CAD build for the part. Positions are in the model's coordinates, mm. A direction names the side the tool comes from. Coordinates: 2 decimals unless noted, no trailing zeros. Order: outer loops, then holes, each group sorted by start corner. A loop starts at its lowest first (then second) coordinate and runs counter-clockwise, first axis right, second up. Notation, with made-up numbers: (-8.5, 65) -> (12.5, 65) arc R25 ccw to (12.5, 86) -> close; hole circle Ø4 at (35.25, 75). An arc over 180 degrees is marked (long way). Use one line per item in the form item = value. Start each with the question number.
from build123d import *

# Parameters (mm, degrees)
SKETCH_1_W          = 20
SKETCH_1_H          = 80
SKETCH_1_R          = 1
EXTRUDE_1_DEPTH     = 1.7
SKETCH_2_W          = 8
SKETCH_2_H          = 10
CUT_EXTRUDE_1_DEPTH = 1
SKETCH_3_W          = 5.4
SKETCH_3_H          = 8.7
EXTRUDE_2_DEPTH     = 2


with BuildPart() as part:
    # 草图1 → 凸台-拉伸1 (new body)
    with BuildSketch(Plane(origin=(0, 0, 0), x_dir=(1, 0, 0), z_dir=(0, 1, 0))):
        Rectangle(SKETCH_1_W, SKETCH_1_H)
        with Locations(Location((-5, 15, 0), (0, 0, 270))):
            Circle(SKETCH_1_R, mode=Mode.SUBTRACT)
        with Locations(Location((-5, -15, 0), (0, 0, 270))):
            Circle(SKETCH_1_R, mode=Mode.SUBTRACT)
        with Locations(Location((5, 35, 0), (0, 0, 270))):
            Circle(SKETCH_1_R, mode=Mode.SUBTRACT)
        with Locations(Location((5, -35, 0), (0, 0, 270))):
            Circle(SKETCH_1_R, mode=Mode.SUBTRACT)
    extrude(amount=EXTRUDE_1_DEPTH)

    # 草图2 → 切除-拉伸1 (cut)
    with BuildSketch(Plane(origin=(0, 1.7, 0), x_dir=(1, 0, 0), z_dir=(0, 1, 0))):
        with Locations((-6, -30)):
            Rectangle(SKETCH_2_W, SKETCH_2_H)
        with Locations((-6, 0)):
            Rectangle(SKETCH_2_W, SKETCH_2_H)
        with Locations((-6, 30)):
            Rectangle(SKETCH_2_W, SKETCH_2_H)
    extrude(amount=-CUT_EXTRUDE_1_DEPTH, mode=Mode.SUBTRACT)

    # 草图3 → 凸台-拉伸2 (add)
    with BuildSketch(Plane.XZ):
        with Locations((7.3, 0)):
            Rectangle(SKETCH_3_W, SKETCH_3_H)
    extrude(amount=EXTRUDE_2_DEPTH)


solid = part.part
1) Cut at A-A on x = -5. Give the cut face in (y, z), then the cut area to 3 significant figures.
2) Two-plate mould, pull along X, no slides. Class faces 4 (the face through (-10, 0.5, 0.6)), 5 (the face through (7, -1, 4.35)), 6 (the face through (-5, 1, -14)): released by +X, released by -X, zero draft, split by the parting line, or undercut.
3) Cut at D-D on z = -27. Give the cut face in (x, y).
4) 3-axis set-ups, long thin cutter, end or side, ignore diameter. For faces 1 (the face through (7, -1, -4.35)), 2 (the face through (-6, 0.7, 0)), 3 (the face through (4.6, -1, 0)): which of +Z, -Z, +X, -X, +Y, -Y reach the whole face in a straight line?
5) Cut at C-C on x = 7.25. Give the cut face in (y, z).
6) Drop flat-ended pins along their axis: P1, Ø2.5, axis at x = -7.5, z = -30, coming from the +Y side; P2, Ø1.6, axis at y = -1, z = 2, coming from the -X side; P3, Ø1.6, axis at x = 6.5, y = -1.5, coming from the -Z side. Give the stop position or say it passes through.
7) Probe L1, parallel to X at y = 0.45, z = -35; L2, parallel to Z at x = 4.25, y = 1; L3, parallel to X at y = 1.15, z = -32.5. List the from-to ranges inside material, lowest first.
8) Cut at B-B on z = -15. Give the cut face in (x, y).
Values follow:
q1.outline = (0, -40) -> (1.7, -40) -> (1.7, -35) -> (0.7, -35) -> (0.7, -25) -> (1.7, -25) -> (1.7, -16) -> (0, -16) -> close; (0, -14) -> (1.7, -14) -> (1.7, -5) -> (0.7, -5) -> (0.7, 5) -> (1.7, 5) -> (1.7, 14) -> (0, 14) -> close; (0, 16) -> (1.7, 16) -> (1.7, 25) -> (0.7, 25) -> (0.7, 35) -> (1.7, 35) -> (1.7, 40) -> (0, 40) -> close
q1.area = 99.2 mm^2
q2.face_4 = released by -X
q2.face_5 = zero draft
q2.face_6 = undercut
q3.outline = (-10, 0) -> (10, 0) -> (10, 1.7) -> (-2, 1.7) -> (-2, 0.7) -> (-10, 0.7) -> close
q4.face_1 = -Z, +X, -X, -Y
q4.face_2 = -X, +Y
q4.face_3 = +Z, -Z, -X, -Y
q5.outline = (-2, -4.35) -> (0, -4.35) -> (0, -40) -> (1.7, -40) -> (1.7, 40) -> (0, 40) -> (0, 4.35) -> (-2, 4.35) -> close
q6.P1 = 0.7
q6.P2 = 4.6
q6.P3 = -4.35
q7.L1 = -10 to 4, 6 to 10
q7.L2 = -40 to -35.66, -34.34 to 34.34, 35.66 to 40
q7.L3 = -2 to 10
q8.outline = (-10, 0) -> (-6, 0) -> (-6, 1.7) -> (-10, 1.7) -> close; (-4, 0) -> (10, 0) -> (10, 1.7) -> (-4, 1.7) -> close
